```python
from build123d import *

# Parameters (mm, degrees)
SKETCH1_W                  = 4
SKETCH1_H                  = 5
BOSS_EXTRUDE1_DEPTH        = 4
SKETCH2_W                  = 4
SKETCH2_H                  = 3
BOSS_EXTRUDE2_DEPTH        = 4
M1_6_CLEARANCE_HOLE1_D     = 1.8
M1_6_CLEARANCE_HOLE1_DEPTH = 4
M1_6_CLEARANCE_HOLE1_TIP   = 0.540774557
M2_CLEARANCE_HOLE1_D       = 2.4
M2_CLEARANCE_HOLE1_DEPTH   = 4
M2_CLEARANCE_HOLE1_TIP     = 0.721032743


with BuildPart() as part:
    # Sketch1 → Boss-Extrude1 (new, symmetric)
    with BuildSketch(Plane(origin=(0, 0, 0), x_dir=(1, 0, 0), z_dir=(0, 1, 0))):
        Rectangle(SKETCH1_W, SKETCH1_H)
    extrude(amount=BOSS_EXTRUDE1_DEPTH, both=True)

    # Sketch2 → Boss-Extrude2 (add)
    with BuildSketch(Plane(origin=(0, 0, -2.5), x_dir=(-1, 0, 0), z_dir=(0, 0, -1))):
        with Locations((0, -2.5)):
            Rectangle(SKETCH2_W, SKETCH2_H)
    extrude(amount=BOSS_EXTRUDE2_DEPTH)

    # M1.6 Clearance Hole1
    with Locations(Plane(origin=(0, -1, 0), x_dir=(1, 0, 0), z_dir=(0, 1, 0))):
        with Locations((0, 4.5)):
            Hole(M1_6_CLEARANCE_HOLE1_D / 2, depth=M1_6_CLEARANCE_HOLE1_DEPTH)
            with Locations((0, 0, -(M1_6_CLEARANCE_HOLE1_DEPTH + M1_6_CLEARANCE_HOLE1_TIP / 2))):  # 118° drill point
                Cone(0, M1_6_CLEARANCE_HOLE1_D / 2, M1_6_CLEARANCE_HOLE1_TIP, mode=Mode.SUBTRACT)

    # M2 Clearance Hole1
    with Locations(Plane.ZY.offset(2)):
        with Locations((0, 0)):
            Hole(M2_CLEARANCE_HOLE1_D / 2, depth=M2_CLEARANCE_HOLE1_DEPTH)
            with Locations((0, 0, -(M2_CLEARANCE_HOLE1_DEPTH + M2_CLEARANCE_HOLE1_TIP / 2))):  # 118° drill point
                Cone(0, M2_CLEARANCE_HOLE1_D / 2, M2_CLEARANCE_HOLE1_TIP, mode=Mode.SUBTRACT)


solid = part.part
```
Geometry: final body of the model. Coordinates: model frame, mm. A direction names the side the tool comes from. Give positions to 0.01 mm unless a question says otherwise; leave off trailing zeros. Write each loop counter-clockwise with the first axis right and the second up, starting at its lowest first coordinate (ties: lowest second). Pieces come first, ordered by that corner, then holes.
1. Pin query (flat end, axial travel): P1, Ø1.2, axis at x = -0.5, z = -4.5, coming from the +Y side. Return the tip coordinate at first contact, or that it passes through.
2. Section query A-A, the plane z = 0. Return loops of the section in (x, y).
3. Line query: probe 1 along X at (y, z) = (-3.3, -4.5); probe 2 along Y at (x, z) = (-0.85, 0); probe 3 along Z at (x, y) = (0, -3.35). Output: solid intervals per line, ascending.
4. Reachability of faces 1 (the flat face through (-2, -1, -1)), 2 (the flat face through (1, -1, -4)) from +Z, -Z, +X, -X, +Y, -Y: full face, straight path, thin tool, end or side. Return the list, or none.
5. Section query C-C, the plane y = 0. Return loops of the section in (x, z).
6. Section query D-D, the plane x = -1.25. Return loops of the section in (y, z), then the cut area to 3 significant figures.
7. Section query B-B, the plane x = 0. Return loops of the section in (y, z).
8. Draft query along X for faces 3 (the flat face through (2, -1, -1)), 4 (the cylindrical face through (0.195, -2.521, -3.621)), 5 (the flat face through (0, 2, -2.5)). Return one class per face: released by +X, released by -X, zero draft, split by the parting line, or undercut.
Computed:
1. P1: stops at y = -1
2. outline: (-2, -4) - (2, -4) - (2, -1.2) - (-2, -1.2) - close; (-2, 1.2) - (2, 1.2) - (2, 4) - (-2, 4) - close
3. probe 1: x = -2 to -0.9, 0.9 to 2
3. probe 2: y = -4 to -1.2, 1.2 to 4
3. probe 3: z = -6.5 to -5.4, -3.6 to 2.5
4. face 1: +Z, -Z, -X, +Y, -Y
4. face 2: -Z, +X, -X, +Y
5. outline: (-2, -2.5) - (2, -2.5) - (2, -1.2) - (-2, -1.2) - close; (-2, 1.2) - (2, 1.2) - (2, 2.5) - (-2, 2.5) - close
6. outline: (-4, -6.5) - (-1, -6.5) - (-1, -2.5) - (4, -2.5) - (4, 2.5) - (-4, 2.5) - close; hole circle Ø2.4 at (0, 0)
6. area: 47.5 mm2
7. outline: (-4, -6.5) - (-1, -6.5) - (-1, -5.4) - (-4, -5.4) - close; (-4, -3.6) - (-1, -3.6) - (-1, -2.5) - (4, -2.5) - (4, 2.5) - (-4, 2.5) - close; hole circle Ø2.4 at (0, 0)
8. face 3: released by +X
8. face 4: undercut
8. face 5: zero draft
